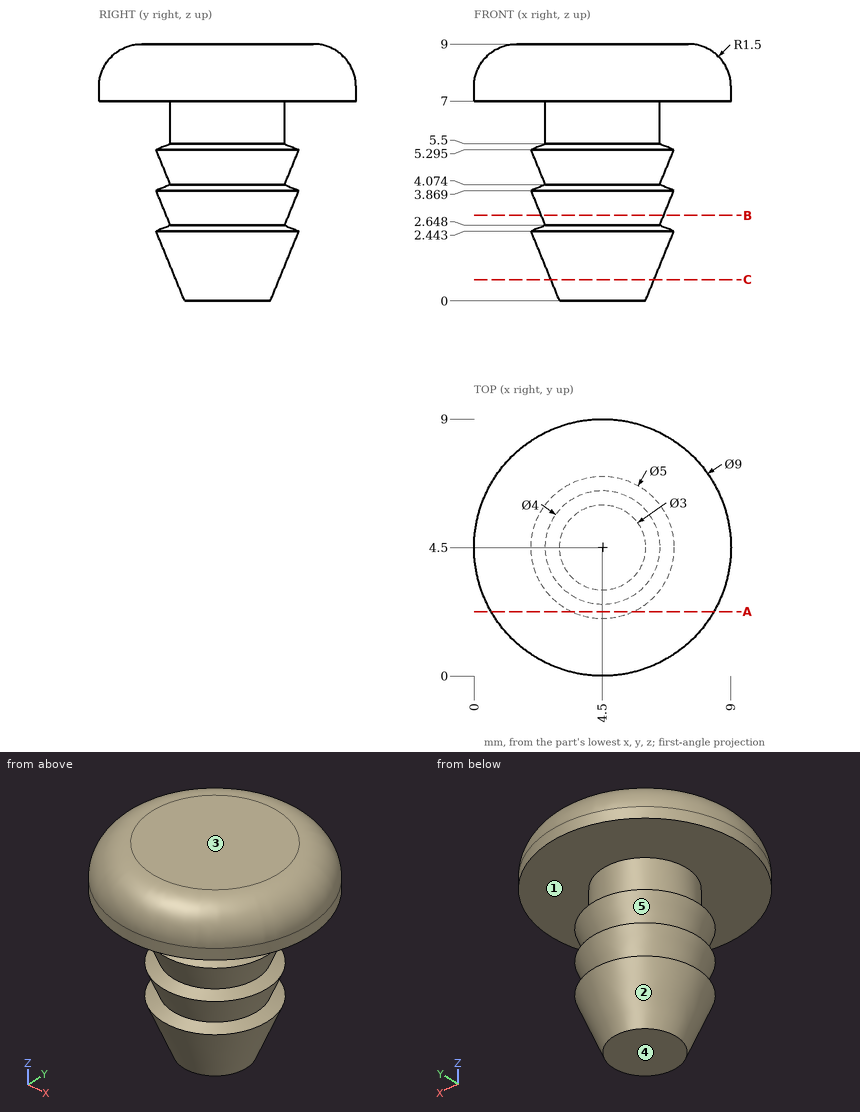
Can you work these out from the drawing? Everything is in mm from the part's minimum corner. A direction names the side the tool comes from. Round coordinates to 2 decimals unless told otherwise and drop trailing zeros. Order: outer loops, then holes, each group sorted by start corner. A loop starts at its lowest first (then second) coordinate and runs counter-clockwise, first axis right, second up. Notation, with made-up numbers: (12.25, 61.25) - (55.25, 61.25) arc R19 ccw to (55.25, 71.25) - close; hole circle Ø2 at (-29.75, 15). An arc over 180 degrees is marked (long way). Answer in a Markdown table with one row per item.
(1) Suppose I cut it at A-A, the plane y = 2.25. Count the separate pieces of the cut face and the enclosed holes in it, plus the area to 3 significant figures.
From the geometry:
| item | result |
|---|---|
| separate pieces | 4 |
| enclosed holes | 0 |
| area | 17.5 mm2 |
(2) Which directions (+Z, -Z, +X, -X, +Y, -Y) give clear straight access to the entire face, cutting with the end or side of a thin tool? Please do the marked faces 1 and 2.
From the geometry:
| item | result |
|---|---|
| face 1 | none |
| face 2 | -Z |
(3) Please list where these lines run through material, in increasing order: L1, parallel to Z at x = 7, y = 3.5; L2, parallel to Z at x = 7.75, y = 6.5; L3, parallel to X at y = 6.5, z = 7.5. Write a range as from..to.
From the geometry:
| item | result |
|---|---|
| L1 | z = 7..9 |
| L2 | z = 7..8.76 |
| L3 | x = 0.47..8.53 |
(4) Suppose I cut it at C-C, the plane z = 0.75. Please give me the cut outline in (x, y), plus the area to 3 significant figures.
From the geometry:
| item | result |
|---|---|
| outline | circle Ø3.61 at (4.5, 4.5) |
| area | 10.3 mm2 |
(5) If we mould it in two halves opening along Z, with no side actions, what happens to the marked faces 3, 4 and 5? For each: released by +Z, released by -Z, zero draft, split by the parting line, or undercut.
From the geometry:
| item | result |
|---|---|
| face 3 | released by +Z |
| face 4 | released by -Z |
| face 5 | undercut |
(6) For P1, Ø3, axis at y = 4.5, z = 2.5, coming from the -X side; P2, Ø1.5, axis at x = 7.5, y = 2, coming from the +Z side; P3, Ø5, axis at y = 7.5, z = 2.5, coming from the +X side, each with a flat end and sliding along its axis, tell me the tip position at first contact or that it passes through.
From the geometry:
| item | result |
|---|---|
| P1 | stops at x = 2 |
| P2 | stops at z = 8.99 |
| P3 | stops at x = 6.95 |
(7) Suppose I cut it at B-B, the plane z = 3. Please give me the cut outline in (x, y).
From the geometry:
| item | result |
|---|---|
| outline | circle Ø4.29 at (4.5, 4.5) |
